The model under review builds one solid part; all positions refer to its coordinate system, in mm. Give positions to 0.01 mm unless a question says otherwise; leave off trailing zeros. Order: outer loops, then holes, each group sorted by start corner. A loop starts at its lowest first (then second) coordinate and runs counter-clockwise, first axis right, second up. Notation, with made-up numbers: (59.25, -2.75) - (67.25, -2.75) arc R31 cw to (67.25, 30.25) - close; hole circle Ø7 at (68.25, 9). An arc over 180 degrees is marked (long way). Write item = value, one per line. Start each with the question number.
1. For P1, Ø2, axis at y = 3.5, z = -2.5, coming from the +X side, flat-tipped, find the tip position at first contact; note if it passes through.
2. We need section B-B, the plane z = -0.75. Give the boundary of the cut face in (x, y), and give its area (3 significant figures).
3. We need section A-A, the plane z = -2.55. Give the boundary of the cut face in (x, y), and give its area (3 significant figures).
4. Wall thickness on probe 1 along X at (y, z) = (0, -1.8); probe 2 along Y at (x, z) = (0, -1.3); probe 3 along Y at (x, z) = (-0.5, -4.5): over which ranges is each line inside the solid? List them lowest first.
from build123d import *

# Parameters (mm, degrees)
BASENUTSKE_R  = 2.1
BASENUT_DEPTH = 5.3


with BuildPart() as part:
    # BaseNutSke → BaseNut (new body)
    with BuildSketch(Plane.XY):
        Polygon((4, 2.309401077), (4, -2.309401077), (0, -4.618802154), (-4, -2.309401077), (-4, 2.309401077), (0, 4.618802154), align=None)
        Circle(BASENUTSKE_R, mode=Mode.SUBTRACT)
    extrude(amount=-BASENUT_DEPTH)

    # Sketch3 → Double-Chamfer (revolve, cut)
    with BuildSketch(Plane(origin=(0, 0, 0), x_dir=(0, 0, -1), z_dir=(1, 0, 0))):
        Polygon((5.3, 4), (4.94273441, 4.618802154), (4.94273441, 14.618802154), (15.3, 14.618802154), (15.3, 4), align=None)
        Polygon((1.46, 14.618802154), (-10, 14.618802154), (-10, 3.8), (0, 3.8), (1.46, 4.618802154), align=None)
    revolve(axis=Axis((0, 0, 0), (0, 0, -1)), mode=Mode.SUBTRACT)

    # Sketch5 → EndChamfer (revolve, cut)
    with BuildSketch(Plane(origin=(0, 0, 0), x_dir=(0, 0, -1), z_dir=(1, 0, 0))):
        Polygon((5.2746, 2.5), (4.966508683, 2.06), (5.3254, 2.06), (5.3254, 2.5), align=None)
        Polygon((-0.0508, 2.5), (0, 2.5), (0.308091317, 2.06), (-0.0508, 2.06), align=None)
    revolve(axis=Axis((0, 0, -25.037505729), (0, 0, -1)), mode=Mode.SUBTRACT)


solid = part.part
Model answer:
q1.P1 = 3.67
q2.outline = (-4, -1.35) arc R4.22 ccw to (-3.17, -2.79) - (-0.83, -4.14) arc R4.22 ccw to (0.83, -4.14) - (3.17, -2.79) arc R4.22 ccw to (4, -1.35) - (4, 1.35) arc R4.22 ccw to (3.17, 2.79) - (0.83, 4.14) arc R4.22 ccw to (-0.83, 4.14) - (-3.17, 2.79) arc R4.22 ccw to (-4, 1.35) - close; hole circle Ø4.2 at (0, 0)
q2.area = 39.7 mm2
q3.outline = (-4, -2.31) - (0, -4.62) - (4, -2.31) - (4, 2.31) - (0, 4.62) - (-4, 2.31) - close; hole circle Ø4.2 at (0, 0)
q3.area = 41.6 mm2
q4.probe_1 = -4 to -2.1, 2.1 to 4
q4.probe_2 = -4.53 to -2.1, 2.1 to 4.53
q4.probe_3 = -4.33 to -2.04, 2.04 to 4.33
